from build123d import *

# Parameters (mm, degrees)
F0_R     = 9.1
F1_DEPTH = 7
F2_R     = 1
F3_R     = 1


with BuildPart() as f1:
    # F0 (on Top) → F1 (new body)
    with BuildSketch(Plane.XY):
        with BuildLine():
            ThreePointArc((-12.1, 0), (0, -12.1), (12.1, 0))
            ThreePointArc((12.1, 0), (0, 12.1), (-12.1, 0))
        make_face()
        Circle(F0_R, mode=Mode.SUBTRACT)
        with BuildLine():
            ThreePointArc((-12.1, 0), (0, 12.1), (12.1, 0))
            Line((12.1, 0), (12.1, 24.9))
            Line((12.1, 24.9), (-12.1, 24.9))
            Line((-12.1, 24.9), (-12.1, 0))
        make_face()
    extrude(amount=F1_DEPTH)

    # F2
    f2_edges = [f1.edges().sort_by_distance(p)[0] for p in [
        (-12.1, 24.9, 3.5),
    ]]
    fillet(f2_edges, radius=F2_R)

    # F3
    f3_edges = [f1.edges().sort_by_distance(p)[0] for p in [
        (12.1, 24.9, 3.5),
    ]]
    fillet(f3_edges, radius=F3_R)


solid = f1.part
Input: part model. Units: mm. Frame: model coordinates. Coordinates: 2 decimals unless noted, no trailing zeros. Order: outer loops, then holes, each group sorted by start corner. A loop starts at its lowest first (then second) coordinate and runs counter-clockwise, first axis right, second up. Notation, with made-up numbers: M 64.25,-38 L 111.25,-38 A23 cw 111.25,-19 Z; hole C -34.5,46 d4. An arc over 180 degrees is marked long. Answer as CSV lines item,"result".
1. First-contact query: P1, Ø3, axis at x = 4.5, y = -6, coming from the -Z side. Flat tip, straight axial feed; report the tip coordinate or a pass-through.
Reported:
P1,"through"
2. Section A-A (x = 0). Return the cut outline in (y, z).
Reported:
outline,"M -12.1,0 L -9.1,0 L -9.1,7 L -12.1,7 Z; M 9.1,0 L 24.9,0 L 24.9,7 L 9.1,7 Z"
3. Section B-B (z = 2.75). Return the cut outline in (x, y).
Reported:
outline,"M -12.1,0 A12.1 ccw 12.1,0 L 12.1,23.9 A1 ccw 11.1,24.9 L -11.1,24.9 A1 ccw -12.1,23.9 Z; hole C 0,0 d18.2"
4. Material intervals for line 1 (Y direction, x = 0, z = 4); line 2 (Y direction, x = 1.5, z = 5.75); line 3 (X direction, y = 4.5, z = 4.5), sorted ascending. Write a range as from..to.
Reported:
line 1,"-12.1..-9.1, 9.1..24.9"
line 2,"-12.01..-8.98, 8.98..24.9"
line 3,"-12.1..-7.91, 7.91..12.1"
5. Pull-direction query (X, two-part tool) for faces 1 (the cylindrical face through (11.799, 24.615, 3.549)), 2 (the cylindrical face through (-0.266, -12.097, 3.451)), 3 (the cylindrical face through (-1.973, -8.884, 3.451)); classes: released by +X, released by -X, zero draft, split by the parting line, or undercut.
Reported:
face 1,"released by +X"
face 2,"split by the parting line"
face 3,"undercut"
6. Section C-C (y = -0.5). Return the cut outline in (x, z).
Reported:
outline,"M -12.09,0 L -9.09,0 L -9.09,7 L -12.09,7 Z; M 9.09,0 L 12.09,0 L 12.09,7 L 9.09,7 Z"
